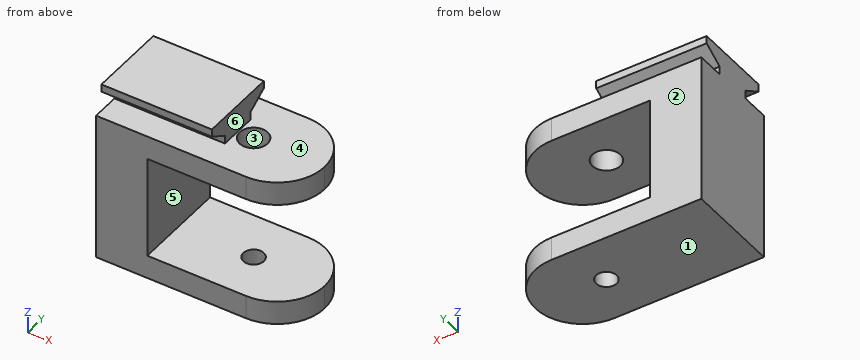
```python
from build123d import *

# Parameters (mm, degrees)
BOSS_EXTRUDE1_DEPTH = 24
SKETCH3_R           = 2.6
CUT_EXTRUDE1_DEPTH  = 60
SKETCH5_R           = 3.55
CUT_EXTRUDE2_DEPTH  = 10
BOSS_EXTRUDE2_DEPTH = 28


with BuildPart() as part:
    # Sketch1 → Boss-Extrude1 (new body)
    with BuildSketch(Plane(origin=(0, 0, 0), x_dir=(1, 0, 0), z_dir=(0, 1, 0))):
        Polygon((0, 0), (50, 0), (50, 6), (13, 6), (13, 32), (50, 32), (50, 38), (0, 38), align=None)
    extrude(amount=BOSS_EXTRUDE1_DEPTH)

    # Sketch3 → Cut-Extrude1 (cut)
    with BuildSketch(Plane(origin=(0, 0, -38), x_dir=(-1, 0, 0), z_dir=(0, 0, -1))):
        with BuildLine():
            Line((-38, 24), (-50, 24))
            Line((-50, 24), (-50, 12))
            ThreePointArc((-50, 12), (-46.485281374, 20.485281374), (-38, 24))
        make_face()
        with BuildLine():
            ThreePointArc((-38, 0), (-46.485281374, 3.514718626), (-50, 12))
            Line((-50, 12), (-50, 0))
            Line((-50, 0), (-38, 0))
        make_face()
        with Locations((-32, 12)):
            Circle(SKETCH3_R)
    extrude(amount=-CUT_EXTRUDE1_DEPTH, mode=Mode.SUBTRACT)

    # Sketch5 → Cut-Extrude2 (cut)
    with BuildSketch(Plane.XY):
        with Locations((32, 12)):
            Circle(SKETCH5_R)
    extrude(amount=-CUT_EXTRUDE2_DEPTH, mode=Mode.SUBTRACT)

    # Sketch7 → Boss-Extrude2 (add)
    with BuildSketch(Plane.ZY):
        Polygon((0, 16.95), (2.1, 16.95), (5.1, 21.95), (7.05, 21.95), (7.05, 2.05), (5.1, 2.05), (2.1, 7.05), (0, 7.05), align=None)
    extrude(amount=-BOSS_EXTRUDE2_DEPTH)


solid = part.part
```
Geometry: final body of the model. Coordinates: model frame, mm. Face numbers are marked on the shaded views. A direction names the side the tool comes from. Round coordinates to 2 decimals unless told otherwise and drop trailing zeros. Loops run counter-clockwise (first coordinate to the right, second up) from the corner with the lowest first, then second, coordinate; pieces in that order, holes last.
Item 1: Section A-A, the plane x = 32. Output: boundary loops of the cut face in (y, z), plus the area to 3 significant figures.
Checked values:
outline: (0, -38) - (9.4, -38) - (9.4, -32) - (0, -32) - close; (0, -6) - (8.45, -6) - (8.45, 0) - (0, 0) - close; (14.6, -38) - (24, -38) - (24, -32) - (14.6, -32) - close; (15.55, -6) - (24, -6) - (24, 0) - (15.55, 0) - close
area: 214 mm2
Item 2: Reachability of the marked faces 4, 5 and 6 from +Z, -Z, +X, -X, +Y, -Y: full face, straight path, thin tool, end or side. Return the list, or none.
Checked values:
face 4: +X
face 5: +X, +Y, -Y
face 6: +Z, +X, +Y, -Y
Item 3: Section D-D, the plane y = 2.75. Output: boundary loops of the cut face in (x, z), plus the area to 3 significant figures.
Checked values:
outline: (0, -38) - (45.64, -38) - (45.64, -32) - (13, -32) - (13, -6) - (45.64, -6) - (45.64, 0) - (0, 0) - close; (0, 4.68) - (28, 4.68) - (28, 7.05) - (0, 7.05) - close
area: 952 mm2
Item 4: Section B-B, the plane z = -35. Output: boundary loops of the cut face in (x, y), plus the area to 3 significant figures.
Checked values:
outline: (0, 0) - (38, 0) arc R12 ccw to (38, 24) - (0, 24) - close; hole circle Ø5.2 at (32, 12)
area: 1,120 mm2
Item 5: Contact query for flat-ended pins moving along their axis: P1, Ø4, axis at y = 13.5, z = -3, coming from the -X side; P2, Ø5, axis at y = 11, z = -20.5, coming from the +X side; P3, Ø0.6, axis at x = 17.5, z = 1, coming from the +Y side; P4, Ø2, axis at x = 8.5, z = 6, coming from the -Y side. Output: stop coordinate, or through.
Checked values:
P1: stops at x = 0
P2: stops at x = 13
P3: stops at y = 16.95
P4: stops at y = 2.05
Item 6: Mould query, pull axis Y, two halves, no side actions, for the marked faces 1, 2 and 3. Classes: released by +Y, released by -Y, zero draft, split by the parting line, or undercut.
Checked values:
face 1: zero draft
face 2: released by +Y
face 3: undercut
Item 7: Line query: L1, parallel to Z at x = 39.5, y = 22.25; L2, parallel to Y at x = 32, z = -1.85; L3, parallel to Z at x = 24.5, y = 14.75. Output: solid intervals per line, ascending.
Checked values:
L1: z = -38 to -32, -6 to 0
L2: y = 0 to 8.45, 15.55 to 24
L3: z = -38 to -32, -6 to 7.05
Item 8: Section C-C, the plane x = 26. Output: boundary loops of the cut face in (y, z).
Checked values:
outline: (0, -38) - (24, -38) - (24, -32) - (0, -32) - close; (0, -6) - (24, -6) - (24, 0) - (16.95, 0) - (16.95, 2.1) - (21.95, 5.1) - (21.95, 7.05) - (2.05, 7.05) - (2.05, 5.1) - (7.05, 2.1) - (7.05, 0) - (0, 0) - close
